from build123d import *

# Parameters (mm, degrees)
F1_DEPTH = 3
F2_D     = 5
F3_D     = 5
F5_DEPTH = 25
F6_DEPTH = 25
F7_DEPTH = 3


with BuildPart() as f1:
    # F0 (on Top) → F1 (new body)
    with BuildSketch(Plane.XY):
        with BuildLine():
            ThreePointArc((7.0710678119, 40), (2.0710678119, 37.9289321881), (0, 32.9289321881))
            Line((0, 32.9289321881), (0, 0))
            Line((0, 0), (0, -107.0710678119))
            ThreePointArc((0, -107.0710678119), (2.0710678119, -112.0710678119), (7.0710678119, -114.1421356237))
            Line((7.0710678119, -114.1421356237), (127.0710678119, -114.1421356237))
            ThreePointArc((127.0710678119, -114.1421356237), (132.0710678119, -112.0710678119), (134.1421356237, -107.0710678119))
            Line((134.1421356237, -107.0710678119), (134.1421356237, 0))
            Line((134.1421356237, 0), (134.1421356237, 32.9289321881))
            ThreePointArc((134.1421356237, 32.9289321881), (132.0710678119, 37.9289321881), (127.0710678119, 40))
            Line((127.0710678119, 40), (7.0710678119, 40))
        make_face()
    extrude(amount=F1_DEPTH)

    # F2 (through all)
    with Locations(Plane(origin=(0, 0, 0), x_dir=(1, 0, 0), z_dir=(0, 0, -1))):
        with Locations((94, 9.0260861005), (32, 9.0260861005)):
            Hole(F2_D / 2)

    # F3 (through all)
    with Locations(Plane(origin=(0, 0, 0), x_dir=(1, 0, 0), z_dir=(0, 0, -1))):
        with Locations((32, 39.5260861005), (94, 39.5260861005)):
            Hole(F3_D / 2)

    # F4 (on face) → F5 (cut)
    with BuildSketch(Plane.XY.offset(3)):
        with BuildLine():
            ThreePointArc((115.5, 0), (113, 2.5), (110.5, 0))
            Line((110.5, 0), (110.5, -48))
            ThreePointArc((110.5, -48), (113, -50.5), (115.5, -48))
            Line((115.5, -48), (115.5, 0))
        make_face()
    extrude(amount=-F5_DEPTH, mode=Mode.SUBTRACT)

    # F4 (on face) → F6 (cut)
    with BuildSketch(Plane.XY.offset(3)):
        with BuildLine():
            ThreePointArc((15.5, 0), (13, 2.5), (10.5, 0))
            Line((10.5, 0), (10.5, -48))
            ThreePointArc((10.5, -48), (13, -50.5), (15.5, -48))
            Line((15.5, -48), (15.5, 0))
        make_face()
    extrude(amount=-F6_DEPTH, mode=Mode.SUBTRACT)

    # F0 (on Top) → F7 (join)
    with BuildSketch(Plane.XY):
        Polygon((67.0710678119, 120), (7.0710678119, 40), (127.0710678119, 40), align=None)
        Polygon((127.0710678119, -114.1421356237), (7.0710678119, -114.1421356237), (67.0710678119, -152.6137888432), align=None)
    extrude(amount=F7_DEPTH)


solid = f1.part
Model file for the job. Use its own axes, mm. Coordinates: 2 decimals unless noted, no trailing zeros. Write each loop counter-clockwise with the first axis right and the second up, starting at its lowest first coordinate (ties: lowest second). Pieces come first, ordered by that corner, then holes. Notation, with made-up numbers: (26, 43) -> (33, 43) arc R10 ccw to (33, 48) -> close; hole circle Ø9 at (9.5, 10). An arc over 180 degrees is marked (long way). One line per item, written item: value. Start each with the question number.
1) Probe probe 1 along X at (y, z) = (-23.5, 2.65); probe 2 along Y at (x, z) = (32, 2.3); probe 3 along Y at (x, z) = (113.5, 0.4). List the from-to ranges inside material, lowest first.
2) Slice it at A-A on y = -20. Write the cut outline in (x, z), then the cut area to 3 significant figures.
3) Slice it at D-D on x = 13. Write the cut outline in (y, z), then the cut area to 3 significant figures.
4) Flat gauge pins, fed straight in: pin 1 Ø3 at (x, y) = (94, -9.03) entering from -Z; pin 2 Ø1.5 at (x, z) = (75, 2.5) entering from +Y. Where does each tip first touch, or does it go through?
5) Slice it at C-C on z = 1.95. Write the cut outline in (x, y).
6) Slice it at B-B on x = 32. Write the cut outline in (y, z).
7) Pull direction Y, two halves, no side cores. Call faces 1 (the face through (96.65, -133.65, 1.48)), 2 (the face through (2.126, 37.984, 1.479)), 3 (the face through (66, -14, 3)), 4 (the face through (34.5, -9.1, 1.5)): +Y half, -Y half, draft (parallel to the pull), parting line (faces both ways), or undercut.
Answers follow:
1. probe 1: 0 to 10.5, 15.5 to 110.5, 115.5 to 134.14
1. probe 2: -130.13 to -42.03, -37.03 to -11.53, -6.53 to 73.24
1. probe 3: -122.84 to -50.45, 2.45 to 58.09
2. outline: (0, 0) -> (10.5, 0) -> (10.5, 3) -> (0, 3) -> close; (15.5, 0) -> (110.5, 0) -> (110.5, 3) -> (15.5, 3) -> close; (115.5, 0) -> (134.14, 0) -> (134.14, 3) -> (115.5, 3) -> close
2. area: 372 mm2
3. outline: (-117.94, 0) -> (-50.5, 0) -> (-50.5, 3) -> (-117.94, 3) -> close; (2.5, 0) -> (47.91, 0) -> (47.91, 3) -> (2.5, 3) -> close
3. area: 339 mm2
4. pin 1: through
4. pin 2: y = 110.43
5. outline: (0, -107.07) arc R7.07 ccw to (7.07, -114.14) -> (67.07, -152.61) -> (127.07, -114.14) arc R7.07 ccw to (134.14, -107.07) -> (134.14, 32.93) arc R7.07 ccw to (127.07, 40) -> (67.07, 120) -> (7.07, 40) arc R7.07 ccw to (0, 32.93) -> close; hole (10.5, -48) arc R2.5 ccw to (15.5, -48) -> (15.5, 0) arc R2.5 ccw to (10.5, 0) -> close; hole circle Ø5 at (32, -39.53); hole circle Ø5 at (32, -9.03); hole circle Ø5 at (94, -39.53); hole circle Ø5 at (94, -9.03); hole (110.5, -48) arc R2.5 ccw to (115.5, -48) -> (115.5, 0) arc R2.5 ccw to (110.5, 0) -> close
6. outline: (-130.13, 0) -> (-42.03, 0) -> (-42.03, 3) -> (-130.13, 3) -> close; (-37.03, 0) -> (-11.53, 0) -> (-11.53, 3) -> (-37.03, 3) -> close; (-6.53, 0) -> (73.24, 0) -> (73.24, 3) -> (-6.53, 3) -> close
7. face 1: -Y half
7. face 2: +Y half
7. face 3: draft
7. face 4: undercut
